Could you check a few things on this model? Use its own coordinates, in mm. Face numbers are marked on the shaded views. A direction names the side the tool comes from. Give positions to 0.01 mm unless a question says otherwise; leave off trailing zeros. Write each loop counter-clockwise with the first axis right and the second up, starting at its lowest first coordinate (ties: lowest second). Pieces come first, ordered by that corner, then holes. Notation, with made-up numbers: (87, 22.25) - (132, 22.25) arc R13 cw to (132, 37.25) - close; hole circle Ø6 at (-29, 86.5). An arc over 180 degrees is marked (long way). Answer as a JSON object with one key per item and string values. Group by question number.
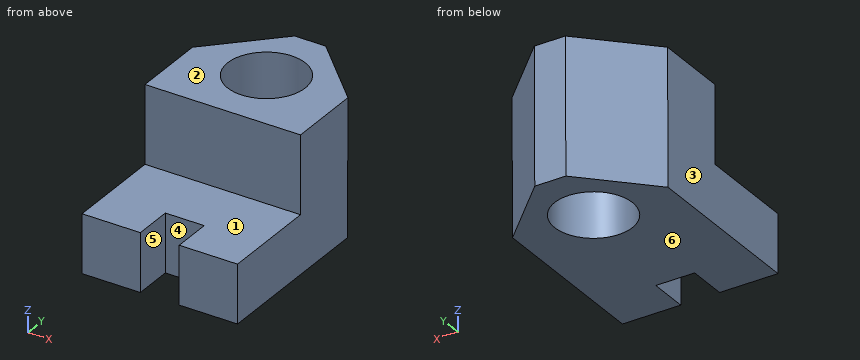
```python
from build123d import *

# Parameters (mm, degrees)
F1_DEPTH = 50.8
F3_D     = 25.4
F4_SIZE  = 20.32
F5_W     = 12.7
F5_H     = 12.7
F6_DEPTH = 0.254
F7_DEPTH = 35.052


with BuildPart() as f1:
    # F0 (on Right) → F1 (new body)
    with BuildSketch(Plane.YZ):
        Polygon((-24.5744947175, 0), (-40.5764947175, 0), (-40.5764947175, -19.05), (35.6235052825, -19.05), (35.8775052825, 25.4), (-8.5724947175, 25.4), (-8.5724947175, 0), align=None)
    extrude(amount=F1_DEPTH)

    # F3 (through all)
    with Locations(Plane.XY.offset(25.4)):
        with Locations((25.4, 13.6525052825)):
            Hole(F3_D / 2)

    # F4
    f4_edges = [f1.edges().sort_by_distance(p)[0] for p in [
        (0, 35.750505, 3.175),
        (50.8, 35.750505, 3.175),
    ]]
    chamfer(f4_edges, length=F4_SIZE)

    # F5 (on face) → F6 (join)
    with BuildSketch(Plane.XY):
        with Locations((25.4, -34.2264947175)):
            Rectangle(F5_W, F5_H)
    extrude(amount=F6_DEPTH)

    # F7 (cut): a face of the model
    f7_faces = [f1.faces().sort_by_distance(p)[0] for p in [
        (25.4, -34.2264947175, 0.254),
    ]]
    extrude(f7_faces, amount=-F7_DEPTH, mode=Mode.SUBTRACT)


solid = f1.part
```
(1) If we mould it in two halves opening along X, with no side actions, what happens to the marked faces 3, 4, 5 and 6? For each: +X half, -X half, draft (parallel to the pull), parting line (faces both ways), or undercut.
(2) Will these pins go through, and if not, where does the flat tip stop? P1, Ø15, axis at x = 25.4, y = 13.65, coming from the +Z side; P2, Ø16, axis at x = 32.5, y = -17, coming from the +Z side; P3, Ø6.5, axis at x = 25, z = -9.5, coming from the -Y side; P4, Ø7.5, axis at x = 32.5, z = 11.5, coming from the -Y side.
(3) I want a section at D-D, the plane x = 34. Please give me the cut outline in (y, z).
(4) I want a section at A-A, the plane x = 25.4. Please give me the cut outline in (y, z).
(5) I need wall thicknesses on L1, parallel to Y at x = 14, z = -2; L2, parallel to Z at x = 4, y = -36; L3, parallel to Y at x = 25.4, z = -9.5. Which ranges of each line are inside material? Lowest first, please.
(6) I want a section at B-B, the plane y = -29. Please give me the cut outline in (x, z), and give its area (3 significant figures).
(7) I want a section at C-C, the plane y = 3.5. Please give me the cut outline in (x, z), and give its area (3 significant figures).
(8) For the marked faces 1 and 2, which set-ups out of +Z, -Z, +X, -X, +Y, -Y let a thin tool reach every point of the face, with its end or its side?
Entries:
{
 "1": {"face 3": "-X half", "face 4": "undercut", "face 5": "undercut", "face 6": "draft"},
 "2": {"P1": "through", "P2": "z = 0", "P3": "y = -27.88", "P4": "y = -8.57"},
 "3": {"outline": "(-40.58, -19.05) - (4.31, -19.05) - (4.31, 25.4) - (-8.57, 25.4) - (-8.57, 0) - (-40.58, 0) - close; (23, -19.05) - (32.1, -19.05) - (32.36, 25.4) - (23, 25.4) - close"},
 "4": {"outline": "(-27.88, -19.05) - (0.95, -19.05) - (0.95, 25.4) - (-8.57, 25.4) - (-8.57, 0) - (-27.88, 0) - close; (26.35, -19.05) - (35.62, -19.05) - (35.88, 25.4) - (26.35, 25.4) - close"},
 "5": {"L1": "-40.58 to 8.06, 19.25 to 29.4", "L2": "-19.05 to 0", "L3": "-27.88 to 0.95, 26.35 to 35.68"},
 "6": {"outline": "(0, -19.05) - (19.05, -19.05) - (19.05, 0) - (0, 0) - close; (31.75, -19.05) - (50.8, -19.05) - (50.8, 0) - (31.75, 0) - close", "area": "726 mm^2"},
 "7": {"outline": "(0, -19.05) - (17.77, -19.05) - (17.77, 25.4) - (0, 25.4) - close; (33.03, -19.05) - (50.8, -19.05) - (50.8, 25.4) - (33.03, 25.4) - close", "area": "1,580 mm^2"},
 "8": {"face 1": "+Z, +X, -X, -Y", "face 2": "+Z, +X, -X, +Y, -Y"}
}
